from build123d import *

# Parameters (mm, degrees)
F0_W      = 146
F0_H      = 148
F0_W_2    = 134
F0_H_2    = 128
F1_DEPTH  = 20
F2_W      = 140
F2_H      = 134
F2_W_2    = 134
F2_H_2    = 128
F3_DEPTH  = 10
F4_W      = 90
F4_H      = 25
F5_DEPTH  = 149.278288
F6_W      = 90
F6_H      = 25
F7_DEPTH  = 148.001
F8_W      = 17
F8_H      = 67
F8_R      = 2.5
F9_DEPTH  = 40
F10_W     = 5
F10_H     = 17
F11_DEPTH = 135.001
F12_W     = 148
F12_H     = 5
F13_DEPTH = 10
F14_R     = 17.5
F15_DEPTH = 7.5
F16_W     = 10
F16_H     = 29
F17_DEPTH = 15
F18_W     = 6
F18_H     = 90
F19_DEPTH = 5
F20_W     = 15
F20_H     = 5
F21_DEPTH = 6
F23_W     = 42.3
F23_H     = 5
F24_DEPTH = 30
F25_R     = 2.25
F26_DEPTH = 5
F27_SIZE  = 4
F28_W     = 40
F28_H     = 5
F29_DEPTH = 25
F31_DEPTH = 42.3
F32_W     = 5
F32_H     = 30
F33_DEPTH = 27.5
F35_DEPTH = 50
F36_R     = 2.25
F37_DEPTH = 10
F39_DEPTH = 5


with BuildPart() as f1:
    # F0 (on Top) → F1 (new body)
    with BuildSketch(Plane.XY):
        with Locations((76.277288, 74)):
            Rectangle(F0_W, F0_H)
        with Locations((76.277288, 74)):
            Rectangle(F0_W_2, F0_H_2, mode=Mode.SUBTRACT)
    extrude(amount=F1_DEPTH)

    # F2 (on face) → F3 (join)
    with BuildSketch(Plane.XY.offset(20)):
        with Locations((76.277288, 74)):
            Rectangle(F2_W, F2_H)
        with Locations((76.277288, 74)):
            Rectangle(F2_W_2, F2_H_2, mode=Mode.SUBTRACT)
    extrude(amount=F3_DEPTH)

    # F4 (on Right) → F5 (cut, through all)
    with BuildSketch(Plane.YZ):
        with Locations((74, 17.5)):
            Rectangle(F4_W, F4_H)
    extrude(amount=F5_DEPTH, mode=Mode.SUBTRACT)

    # F6 (on Front) → F7 (cut, through all)
    with BuildSketch(Plane.XZ):
        with Locations((76.277288, 17.5)):
            Rectangle(F6_W, F6_H)
    extrude(amount=-F7_DEPTH, mode=Mode.SUBTRACT)

    # F8 (on face) → F9 (join)
    with BuildSketch(Plane.XZ):
        with Locations((22.777288, 33.5)):
            Rectangle(F8_W, F8_H)
        with Locations((22.777288, 58.5)):
            Circle(F8_R, mode=Mode.SUBTRACT)
        with Locations((129.777288, 33.5)):
            Rectangle(F8_W, F8_H)
        with Locations((129.777288, 58.5)):
            Circle(F8_R, mode=Mode.SUBTRACT)
    extrude(amount=F9_DEPTH)

    # F10 (on face) → F11 (cut, through all)
    with BuildSketch(Plane(origin=(14.277288, 0, 0), x_dir=(0, -1, 0), z_dir=(-1, 0, 0))):
        Polygon((0, 67), (0, 20), (30, 50), (30, 67), align=None)
        with Locations((37.5, 58.5)):
            Rectangle(F10_W, F10_H)
        Polygon((40, 40), (0, 0), (40, 0), align=None)
    extrude(amount=-F11_DEPTH, mode=Mode.SUBTRACT)

    # F12 (on face) → F13 (join)
    with BuildSketch(Plane(origin=(3.277288, 0, 0), x_dir=(0, -1, 0), z_dir=(-1, 0, 0))):
        with Locations((-74, 2.5)):
            Rectangle(F12_W, F12_H)
    extrude(amount=F13_DEPTH)

    # F14 (on face) → F15 (join)
    with BuildSketch(Plane(origin=(-6.722712, 0, 0), x_dir=(0, -1, 0), z_dir=(-1, 0, 0))):
        with BuildLine():
            Line((-148, 135), (-148, 0))
            Line((-148, 0), (-98, 0))
            Line((-98, 0), (-98, 135))
            ThreePointArc((-98, 135), (-123, 160), (-148, 135))
        make_face()
        with Locations((-123, 135)):
            Circle(F14_R, mode=Mode.SUBTRACT)
    extrude(amount=F15_DEPTH)

    # F16 (on face) → F17 (join, through all)
    with BuildSketch(Plane.XY.offset(5)):
        with Locations((-1.722712, 133.5)):
            Rectangle(F16_W, F16_H)
    extrude(amount=F17_DEPTH)

    # F18 (on face) → F19 (join)
    with BuildSketch(Plane.XY.offset(5)):
        with Locations((146.277288, 74)):
            Rectangle(F18_W, F18_H)
    extrude(amount=F19_DEPTH)

    # F20 (on face) → F21 (cut, through all)
    with BuildSketch(Plane.YZ.offset(149.277288)):
        with Locations((36.5, 2.5)):
            Rectangle(F20_W, F20_H)
        with Locations((111.5, 2.5)):
            Rectangle(F20_W, F20_H)
    extrude(amount=-F21_DEPTH, mode=Mode.SUBTRACT)

    # F23 (on face) → F24 (join)
    with BuildSketch(Plane(origin=(-6.722712, 0, 0), x_dir=(0, -1, 0), z_dir=(-1, 0, 0))):
        with Locations((-21.15, 2.5)):
            Rectangle(F23_W, F23_H)
    extrude(amount=F24_DEPTH)

    # F25 (on face) → F26 (join)
    with BuildSketch(Plane(origin=(-36.722712, 0, 0), x_dir=(0, -1, 0), z_dir=(-1, 0, 0))):
        with BuildLine():
            Line((-42.3, 75), (-42.3, 0))
            Line((-42.3, 0), (0, 0))
            Line((0, 0), (0, 75))
            Line((0, 75), (-11.3, 75))
            Line((-11.3, 75), (-11.3, 61.54594))
            ThreePointArc((-11.3, 61.54594), (-21.15, 41.35), (-31, 61.54594))
            Line((-31, 61.54594), (-31, 75))
            Line((-31, 75), (-42.3, 75))
        make_face()
        with Locations((-36.65, 38.35)):
            Circle(F25_R, mode=Mode.SUBTRACT)
        with Locations((-36.65, 69.35)):
            Circle(F25_R, mode=Mode.SUBTRACT)
        with Locations((-5.65, 38.35)):
            Circle(F25_R, mode=Mode.SUBTRACT)
        with Locations((-5.65, 69.35)):
            Circle(F25_R, mode=Mode.SUBTRACT)
    extrude(amount=F26_DEPTH)

    # F27
    f27_edges = [f1.edges().sort_by_distance(p)[0] for p in [
        (-39.222712, 42.3, 75),
        (-39.222712, 0, 75),
    ]]
    chamfer(f27_edges, length=F27_SIZE)

    # F28 (on face) → F29 (join)
    with BuildSketch(Plane.XY.offset(5)):
        with Locations((-16.722712, 39.8)):
            Rectangle(F28_W, F28_H)
        with Locations((-16.722712, 2.5)):
            Rectangle(F28_W, F28_H)
    extrude(amount=F29_DEPTH)

    # F30 (on face) → F31 (cut, through all)
    with BuildSketch(Plane.XZ):
        Polygon((3.277288, 30), (-36.722712, 30), (3.277288, 5), align=None)
    extrude(amount=-F31_DEPTH, mode=Mode.SUBTRACT)

    # F32 (on face) → F33 (join, through all)
    with BuildSketch(Plane(origin=(-14.222712, 0, 0), x_dir=(0, -1, 0), z_dir=(-1, 0, 0))):
        with Locations((-145.5, 15)):
            Rectangle(F32_W, F32_H)
        with Locations((-100.5, 15)):
            Rectangle(F32_W, F32_H)
    extrude(amount=F33_DEPTH)

    # F34 (on face) → F35 (cut, through all)
    with BuildSketch(Plane(origin=(0, 148, 0), x_dir=(-1, 0, 0), z_dir=(0, 1, 0))):
        Polygon((41.722712, 5), (41.722712, 30), (14.222712, 30), align=None)
    extrude(amount=-F35_DEPTH, mode=Mode.SUBTRACT)

    # F36 (on Top) → F37 (join)
    with BuildSketch(Plane.XY):
        with BuildLine():
            Line((31.277288, 10), (31.277288, 21.5))
            ThreePointArc((31.277288, 21.5), (29.080588, 26.803301), (23.777288, 29))
            Line((23.777288, 29), (9.277288, 29))
            Line((9.277288, 29), (9.277288, 10))
            Line((9.277288, 10), (31.277288, 10))
        make_face()
        with Locations((23.777288, 21.5)):
            Circle(F36_R, mode=Mode.SUBTRACT)
        with BuildLine():
            Line((121.277288, 21.5), (121.277288, 10))
            Line((121.277288, 10), (143.277288, 10))
            Line((143.277288, 10), (143.277288, 29))
            Line((143.277288, 29), (128.777288, 29))
            ThreePointArc((128.777288, 29), (123.473987, 26.803301), (121.277288, 21.5))
        make_face()
        with Locations((128.777288, 21.5)):
            Circle(F36_R, mode=Mode.SUBTRACT)
        with BuildLine():
            Line((143.277288, 138), (121.277288, 138))
            Line((121.277288, 138), (121.277288, 126.5))
            ThreePointArc((121.277288, 126.5), (123.473987, 121.196699), (128.777288, 119))
            Line((128.777288, 119), (143.277288, 119))
            Line((143.277288, 119), (143.277288, 138))
        make_face()
        with Locations((128.777288, 126.5)):
            Circle(F36_R, mode=Mode.SUBTRACT)
        with BuildLine():
            Line((31.277288, 126.5), (31.277288, 138))
            Line((31.277288, 138), (9.277288, 138))
            Line((9.277288, 138), (9.277288, 119))
            Line((9.277288, 119), (23.777288, 119))
            ThreePointArc((23.777288, 119), (29.080588, 121.196699), (31.277288, 126.5))
        make_face()
        with Locations((23.777288, 126.5)):
            Circle(F36_R, mode=Mode.SUBTRACT)
    extrude(amount=F37_DEPTH)

    # F38 (on face) → F39 (cut)
    with BuildSketch(Plane(origin=(0, 0, 0), x_dir=(1, 0, 0), z_dir=(0, 0, -1))):
        Polygon((25.798014, -18), (21.756562, -18), (19.735836, -21.5), (21.756562, -25), (25.798014, -25), (27.818739, -21.5), align=None)
        Polygon((126.756562, -18), (124.735836, -21.5), (126.756562, -25), (130.798014, -25), (132.818739, -21.5), (130.798014, -18), align=None)
        Polygon((126.756562, -130), (130.798014, -130), (132.818739, -126.5), (130.798014, -123), (126.756562, -123), (124.735836, -126.5), align=None)
        Polygon((25.798014, -130), (27.818739, -126.5), (25.798014, -123), (21.756562, -123), (19.735836, -126.5), (21.756562, -130), align=None)
    extrude(amount=-F39_DEPTH, mode=Mode.SUBTRACT)


solid = f1.part
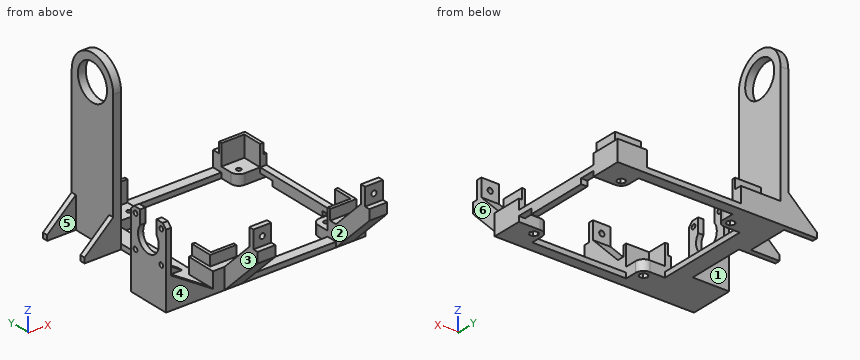
The model under review builds one solid part; all positions refer to its coordinate system, in mm. Face numbers are marked on the shaded views. A direction names the side the tool comes from. Give positions to 0.01 mm unless a question says otherwise; leave off trailing zeros. Order: outer loops, then holes, each group sorted by start corner. A loop starts at its lowest first (then second) coordinate and runs counter-clockwise, first axis right, second up. Notation, with made-up numbers: M 35,88.25 L 49,88.25 A34 cw 49,124.25 Z; hole C 1.25,36.25 d5. An arc over 180 degrees is marked long. Use one line per item in the form item = value. Start each with the question number.
Item 1: We need section C-C on x = 41.5. Give the boundary of the cut face in (y, z), plus the area to 3 significant figures.
Item 2: Insertion check: pin 1 Ø17 at (x, z) = (-10, 42) entering from -Y; pin 2 Ø12 at (x, z) = (1.5, 141) entering from +Y; pin 3 Ø2.5 at (x, y) = (131.5, -33) entering from +Z; pin 4 Ø5.5 at (y, z) = (124, 24) entering from -X. Each pin has a flat end and moves straight along its axis. Give the tip position at first contact, or say it passes through.
Item 3: We need section D-D on z = 58.5. Give the boundary of the cut face in (x, y), plus the area to 3 significant figures.
Item 4: We need section A-A on z = 33. Give the boundary of the cut face in (x, y).
Item 5: For the marked faces 4, 5 and 6, list the 3-axis set-ups (+Z, -Z, +X, -X, +Y, -Y) from which the entire face can be reached by the end or side of a thin tool; tool diameter is ignored.
Item 6: The part is to be moulded in two halves that separate along X. For the marked faces 1, 2 and 3, say which applies: pulls with the +X half, pulls with the -X half, needs draft (parallel to the pull), parting line crosses it, or undercut.
Item 7: We need section B-B on y = -13.5. Give the boundary of the cut face in (x, z), plus the area to 3 significant figures.
Item 8: To check wall thickness, follow line 1 along X through (y, z) = (126.5, 7.15); line 2 along X through (y, z) = (126, 6); line 3 along Y through (x, z) = (0, 11.5). State the ranges of each line that lie inside material, in increasing order. Write a range as from..to.
Completed:
q1.outline = M 0,0 L 10,0 L 10,5 L 0,5 Z; M 138,0 L 148,0 L 148,5 L 138,5 Z
q1.area = 100 mm²
q2.pin_1 = 98
q2.pin_2 = through
q2.pin_3 = 67
q2.pin_4 = -14.22
q3.outline = M -41.72,0 L -36.72,0 L -36.72,9.55 L -41.72,9.55 Z; M -41.72,32.75 L -36.72,32.75 L -36.72,42.3 L -41.72,42.3 Z; M -14.22,98 L -6.72,98 L -6.72,148 L -14.22,148 Z; M 14.28,-35 L 20.28,-35 L 20.28,-30 L 14.28,-30 Z; M 25.28,-35 L 31.28,-35 L 31.28,-30 L 25.28,-30 Z; M 121.28,-35 L 127.28,-35 L 127.28,-30 L 121.28,-30 Z; M 132.28,-35 L 138.28,-35 L 138.28,-30 L 132.28,-30 Z
q3.area = 590 mm²
q4.outline = M -41.72,0 L -36.72,0 L -36.72,42.3 L -41.72,42.3 Z; M -14.22,98 L -6.72,98 L -6.72,148 L -14.22,148 Z; M 14.28,-33 L 31.28,-33 L 31.28,-13 L 14.28,-13 Z; M 121.28,-33 L 138.28,-33 L 138.28,-13 L 121.28,-13 Z
q5.face_4 = +Z, -Z, -X, -Y
q5.face_5 = +Z, -Z, -X
q5.face_6 = +Z, -Z, +X, -Y
q6.face_1 = needs draft
q6.face_2 = undercut
q6.face_3 = pulls with the -X half
q7.outline = M 14.28,13.5 L 31.28,13.5 L 31.28,33.5 L 14.28,33.5 Z; M 121.28,13.5 L 138.28,13.5 L 138.28,33.5 L 121.28,33.5 Z
q7.area = 680 mm²
q8.line_1 = -14.22..21.53, 26.03..31.28, 121.28..126.53, 131.03..149.28
q8.line_2 = -14.22..21.58, 25.97..31.26, 121.29..126.58, 130.97..149.28
q8.line_3 = 119..148
